Input: part model. Units: mm. Frame: model coordinates. A direction names the side the tool comes from. Coordinates: 2 decimals unless noted, no trailing zeros. Write each loop counter-clockwise with the first axis right and the second up, starting at its lowest first coordinate (ties: lowest second). Pieces come first, ordered by that corner, then holes. Notation, with made-up numbers: (13, 53.5) - (45, 53.5) arc R14 cw to (45, 78.5) - close; hole circle Ø4 at (-20, 49). An arc over 180 degrees is marked (long way). Use a Markdown table: item, result. Add a question column.
Q1. Section query A-A (x = 15). Return the cut outline in (y, z), then the cut area to 3 significant figures.
Q2. Material intervals for probe 1 along Y at (x, z) = (-15, 2.25); probe 2 along X at (y, z) = (116, 3); probe 3 along X at (y, z) = (239, 4), sorted ascending. Write a range as from..to.
Q3. Section query C-C (y = 240). Return the cut outline in (x, z).
Q4. Section query D-D (x = -119.5). Return the cut outline in (y, z), then the cut area to 3 significant figures.
Q5. Section query B-B (y = 15). Return the cut outline in (x, z).
Q6. Mould query, pull axis X, two halves, no side actions, for faces 3 (the face through (107.28, 174.15, 3.13)), 4 (the face through (127.56, 96.4, 3.13)), 5 (the face through (-112.53, 232.22, 3.13)), 6 (the face through (147.15, 194.46, 3.13)). Classes: released by +X, released by -X, zero draft, split by the parting line, or undercut.
Q7. Pin query (flat end, axial travel): P1, Ø6.5, axis at x = -15, y = 240, coming from the +Z side; P2, Ø1.5, axis at x = -15.5, z = 3.5, coming from the -Y side; P3, Ø3, axis at x = 76, z = 3, coming from the -Y side; P4, Ø2, axis at y = 192, z = 5, coming from the -X side. Return the tip coordinate at first contact, or that it passes through.
Q8. Set-up query: faces 1 (the face through (-14.09, 255.9, 3.13)), 2 (the face through (-109.5, 83, 3)). Return all of +Z, -Z, +X, -X, +Y, -Y with unobstructed straight access to the full face (end or side cutting, diameter ignored); none if empty.
from build123d import *

# Parameters (mm, degrees)
SALIENTE_EXTRUIR1_DEPTH      = 6.35
TALADRO_DE_MARGEN_PARA_M81_D = 8.4


with BuildPart() as part:
    # Croquis1 → Saliente-Extruir1 (new body)
    with BuildSketch(Plane.XY):
        with BuildLine():
            Line((-63.536796564, 221.213203436), (-100.713203436, 184.036796564))
            ThreePointArc((-100.713203436, 184.036796564), (-107.216385975, 174.3040961), (-109.5, 162.823593129))
            Line((-109.5, 162.823593129), (-109.5, 0))
            Line((-109.5, 0), (-149.5, 0))
            Line((-149.5, 0), (-149.5, 182.823593129))
            ThreePointArc((-149.5, 182.823593129), (-147.216385975, 194.3040961), (-140.713203436, 204.036796564))
            Line((-140.713203436, 204.036796564), (-83.536796564, 261.213203436))
            ThreePointArc((-83.536796564, 261.213203436), (-73.8040961, 267.716385975), (-62.323593129, 270))
            Line((-62.323593129, 270), (62.323593129, 270))
            ThreePointArc((62.323593129, 270), (73.8040961, 267.716385975), (83.536796564, 261.213203436))
            Line((83.536796564, 261.213203436), (140.713203436, 204.036796564))
            ThreePointArc((140.713203436, 204.036796564), (147.216385975, 194.3040961), (149.5, 182.823593129))
            Line((149.5, 182.823593129), (149.5, 0))
            Line((149.5, 0), (109.5, 0))
            Line((109.5, 0), (109.5, 162.823593129))
            ThreePointArc((109.5, 162.823593129), (107.216385975, 174.3040961), (100.713203436, 184.036796564))
            Line((100.713203436, 184.036796564), (63.536796564, 221.213203436))
            ThreePointArc((63.536796564, 221.213203436), (53.8040961, 227.716385975), (42.323593129, 230))
            Line((42.323593129, 230), (-42.323593129, 230))
            ThreePointArc((-42.323593129, 230), (-53.8040961, 227.716385975), (-63.536796564, 221.213203436))
        make_face()
    extrude(amount=SALIENTE_EXTRUIR1_DEPTH)

    # Taladro de margen para M81 (through all)
    with Locations(Plane.XY.offset(6.35)):
        with Locations((-119.5, 15), (-139.5, 15), (0, 15), (139.5, 15), (-15, 260), (-15, 240), (15, 240), (15, 260), (-129.5, 100.125), (-97.125, 217.625), (129.5, 100.125), (97.125, 217.625), (119.5, 15)):
            Hole(TALADRO_DE_MARGEN_PARA_M81_D / 2)


solid = part.part
Values follow:
| question | item | result |
|---|---|---|
| 1 | outline | (230, 0) - (235.8, 0) - (235.8, 6.35) - (230, 6.35) - close; (244.2, 0) - (255.8, 0) - (255.8, 6.35) - (244.2, 6.35) - close; (264.2, 0) - (270, 0) - (270, 6.35) - (264.2, 6.35) - close |
| 1 | area | 147 mm2 |
| 2 | probe 1 | 230..235.8, 244.2..255.8, 264.2..270 |
| 2 | probe 2 | -149.5..-109.5, 109.5..149.5 |
| 2 | probe 3 | -105.75..-19.08, -10.92..10.92, 19.08..105.75 |
| 3 | outline | (-104.75, 0) - (-19.2, 0) - (-19.2, 6.35) - (-104.75, 6.35) - close; (-10.8, 0) - (10.8, 0) - (10.8, 6.35) - (-10.8, 6.35) - close; (19.2, 0) - (104.75, 0) - (104.75, 6.35) - (19.2, 6.35) - close |
| 4 | outline | (0, 0) - (10.8, 0) - (10.8, 6.35) - (0, 6.35) - close; (19.2, 0) - (225.25, 0) - (225.25, 6.35) - (19.2, 6.35) - close |
| 4 | area | 1,380 mm2 |
| 5 | outline | (-149.5, 0) - (-143.7, 0) - (-143.7, 6.35) - (-149.5, 6.35) - close; (-135.3, 0) - (-123.7, 0) - (-123.7, 6.35) - (-135.3, 6.35) - close; (-115.3, 0) - (-109.5, 0) - (-109.5, 6.35) - (-115.3, 6.35) - close; (109.5, 0) - (115.3, 0) - (115.3, 6.35) - (109.5, 6.35) - close; (123.7, 0) - (135.3, 0) - (135.3, 6.35) - (123.7, 6.35) - close; (143.7, 0) - (149.5, 0) - (149.5, 6.35) - (143.7, 6.35) - close |
| 6 | face 3 | undercut |
| 6 | face 4 | undercut |
| 6 | face 5 | released by -X |
| 6 | face 6 | released by +X |
| 7 | P1 | through |
| 7 | P2 | y = 230 |
| 7 | P3 | y = 207.25 |
| 7 | P4 | x = -148.36 |
| 8 | face 1 | +Z, -Z |
| 8 | face 2 | +Z, -Z, -Y |
